Input: part model. Units: mm. Frame: model coordinates. A direction names the side the tool comes from. Coordinates: 2 decimals unless noted, no trailing zeros. Loops run counter-clockwise (first coordinate to the right, second up) from the corner with the lowest first, then second, coordinate; pieces in that order, holes last. Notation, with made-up numbers: (-11.75, -36) -> (19.25, -36) arc R31 ccw to (19.25, -5) -> close; hole circle Ø2 at (52, 20). An arc over 180 degrees is marked (long way). Answer as a JSON object with one key per item and string values.
from build123d import *

# Parameters (mm, degrees)
SKIZZE5_OUTSIDE_W               = 34.244
SKIZZE5_OUTSIDE_H               = 34.244
SKIZZE5_OUTSIDE_W_2             = 8
SKIZZE5_OUTSIDE_H_2             = 20
SCHNITT_LINEAR_AUSTRAGEN1_DEPTH = 15
M3_GEWINDEBOHRUNG1_D            = 2.5
M3_GEWINDEBOHRUNG1_DEPTH        = 8.5
M3_GEWINDEBOHRUNG1_TIP          = 0.751075774


with BuildPart() as part:
    # Skizze2 one side → Rotation1 (revolve)
    with BuildSketch(Plane.XY):
        with BuildLine():
            Line((-4, 0), (4, 0))
            ThreePointArc((4, 0), (0, 4), (-4, 0))
        make_face()
        Polygon((-63, 0), (15, 0), (15, 7.711324865), (14.5, 8), (-63, 8), align=None)
    revolve(axis=Axis((15, 0, 0), (-1, 0, 0)))

    # Skizze3 → Schnitt-Rotation1 (revolve, cut)
    with BuildSketch(Plane(origin=(0, 0, 0), x_dir=(1, 0, 0), z_dir=(0, 1, 0))):
        Polygon((-4.866025404, 8), (-4, 6.5), (-4, -6.5), (-4.866025404, -8), (0, -8), (0, 8), align=None)
    revolve(axis=Axis((0, 0, 8), (0, 0, -1)), mode=Mode.SUBTRACT)

    # Skizze5 outside → Schnitt-Linear austragen1 (cut)
    with BuildSketch(Plane.ZY.offset(63)):
        Rectangle(SKIZZE5_OUTSIDE_W, SKIZZE5_OUTSIDE_H)
        Rectangle(SKIZZE5_OUTSIDE_W_2, SKIZZE5_OUTSIDE_H_2, mode=Mode.SUBTRACT)
    extrude(amount=-SCHNITT_LINEAR_AUSTRAGEN1_DEPTH, mode=Mode.SUBTRACT)

    # M3 Gewindebohrung1
    with Locations(Plane.ZY.offset(63)):
        with Locations((0, 0)):
            Hole(M3_GEWINDEBOHRUNG1_D / 2, depth=M3_GEWINDEBOHRUNG1_DEPTH)
            with Locations((0, 0, -(M3_GEWINDEBOHRUNG1_DEPTH + M3_GEWINDEBOHRUNG1_TIP / 2))):  # 118° drill point
                Cone(0, M3_GEWINDEBOHRUNG1_D / 2, M3_GEWINDEBOHRUNG1_TIP, mode=Mode.SUBTRACT)


solid = part.part
1. Section query A-A (x = -56). Return loops of the section in (y, z), plus the area to 3 significant figures.
Reply:
{"outline": "(-6.93, -4) -> (6.93, -4) arc R8 ccw to (6.93, 4) -> (-6.93, 4) arc R8 ccw to start; hole circle Ø2.5 at (0, 0)", "area": "118 mm2"}
2. Pin query (flat end, axial travel): P1, Ø4, axis at x = -24, z = 6, coming from the +Y side; P2, Ø7, axis at x = -57, y = 3.5, coming from the -Z side; P3, Ø1.2, axis at y = 0, z = -6.5, coming from the -X side. Return the tip coordinate at first contact, or that it passes through.
Reply:
{"P1": "stops at y = 6.93", "P2": "stops at z = -4", "P3": "stops at x = -48"}
3. Mould query, pull axis X, two halves, no side actions, for faces 1 (the face through (-53.88, -0.21, -0.05)), 2 (the face through (-56, 0, 4)), 3 (the face through (0.867, -3.905, 0.091)), 4 (the face through (15, 0, 0)). Classes: pulls with the +X half, pulls with the -X half, needs draft (parallel to the pull), parting line crosses it, or undercut.
Reply:
{"face 1": "pulls with the -X half", "face 2": "needs draft", "face 3": "undercut", "face 4": "pulls with the +X half"}
4. Section query C-C (x = -22.5). Return loops of the section in (y, z), plus the area to 3 significant figures.
Reply:
{"outline": "circle Ø16 at (0, 0)", "area": "201 mm2"}
5. Section query B-B (x = 0). Return loops of the section in (y, z), plus the area to 3 significant figures.
Reply:
{"outline": "(-4.18, -6.82) -> (-4, -6.5) -> (-4, 6.5) -> (-4.18, 6.82) arc R8 ccw to start; (4, -6.5) -> (4.18, -6.82) arc R8 ccw to (4.18, 6.82) -> (4, 6.5) -> close", "area": "78.5 mm2"}
6. Line query: line 1 along Z through (x, y) = (-59, 0); line 2 along Y through (x, z) = (-61.25, 0); line 3 along X through (y, z) = (1.5, 7). Output: solid intervals per line, ascending.
Reply:
{"line 1": "z = -4 to -1.25, 1.25 to 4", "line 2": "y = -8 to -1.25, 1.25 to 8", "line 3": "x = -48 to -4.02, 4.02 to 15"}
7. Access query for faces 5 (the face through (-16.18, 7.63, -2.4)), 6 (the face through (-58.69, -1.22, 0.27)), 7 (the face through (-63, 2, 0)), 8 (the face through (-48, 0, 6)), 9 (the face through (-56, 0, -4)). Directions: +Z, -Z, +X, -X, +Y, -Y. A direction counts if a zero-diameter tool reaches every point of the face in a straight line with its end or side. Return the directions, or none.
Reply:
{"face 5": "+X, -X", "face 6": "-X", "face 7": "+Z, -Z, -X, +Y, -Y", "face 8": "+Z, -X, +Y, -Y", "face 9": "-Z, -X, +Y, -Y"}
